```python
from build123d import *

# Parameters (mm, degrees)
F1_DEPTH = 6.5
F3_D     = 8.3


with BuildPart() as f1:
    # F0 (on Top) → F1 (new body)
    with BuildSketch(Plane.XY):
        Polygon((120, -32.1539030917), (0, 0), (-120, -32.1539030917), (-120, -156.3870447409), (0, -124.2331416492), (120, -156.3870447409), align=None)
    extrude(amount=F1_DEPTH)

    # F3 (through all)
    with Locations(Plane.XY.offset(6.5)):
        with Locations((-90, -44.820950927), (-41.7037086855, -31.8799986719), (-79.6472381959, -83.4579839786), (-31.3509468814, -70.5170317234), (-69.2944763918, -122.0950170301), (41.7037086855, -31.8799986719), (90, -44.820950927), (79.6472381959, -83.4579839786), (69.2944763918, -122.0950170301), (31.3509468814, -70.5170317234)):
            Hole(F3_D / 2)


solid = f1.part
```
Verification items for the finished model (mm, model axes). A direction names the side the tool comes from. Give positions to 0.01 mm unless a question says otherwise; leave off trailing zeros. Order: outer loops, then holes, each group sorted by start corner. A loop starts at its lowest first (then second) coordinate and runs counter-clockwise, first axis right, second up. Notation, with made-up numbers: M 13.5,40.25 L 30.5,40.25 A18 cw 30.5,55.25 Z; hole C 49,-10.75 d9. An arc over 180 degrees is marked long. Answer in a Markdown table with one row per item. Add a question column.
Item 1: Tool access check on faces 1 (the flat face through (59.16, -140.085, 3.204)), 2 (the cylindrical face through (-37.558, -31.698, 3.204)). Record the directions out of +Z, -Z, +X, -X, +Y, -Y that give a thin tool (end or side, any length) a straight path to the whole face; none if there is none.
Item 2: Section check C-C, the plane x = -59. Enter the section's corners in (y, z), and give its area (3 significant figures).
Item 3: Section check A-A, the plane x = -90.5. Enter the section's corners in (y, z), and give its area (3 significant figures).
Item 4: Scan lines: probe 1 along X at (y, z) = (-74, 4.75); probe 2 along X at (y, z) = (-124, 0.5); probe 3 along Y at (x, z) = (-73, 6). Record each from-to range of solid material in increasing order. Write a range as from..to.
Item 5: Section check B-B, the plane z = 3.5. State how many separate pieces and enclosed holes the cut face has, and give its area (3 significant figures).
Item 6: Mould release check, pull along X, two halves, no side actions. Record for faces 3 (the cylindrical face through (29.44, -74.2, 3.2)), 4 (the flat face through (-59.16, -15.85, 3.2)), 5 (the flat face through (-2, -77, 6.5)): released by +X, released by -X, zero draft, split by the parting line, or undercut.
Item 7: Gauge pin test, flat ends, axial feed: pin 1 (7.5 mm diameter, centred on x = 69.29, y = -122.1, fed in from -Z); pin 2 (1 mm diameter, centred on x = -50.5, z = 2.5, fed in from -Y). Record the tip position at first contact, or that the pin passes through.
Filled sheet:
| question | item | result |
|---|---|---|
| 1 | face 1 | +Z, -Z, -Y |
| 1 | face 2 | +Z, -Z |
| 2 | outline | M -140.04,0 L -15.81,0 L -15.81,6.5 L -140.04,6.5 Z |
| 2 | area | 808 mm^2 |
| 3 | outline | M -148.48,0 L -48.94,0 L -48.94,6.5 L -148.48,6.5 Z; M -40.7,0 L -24.25,0 L -24.25,6.5 L -40.7,6.5 Z |
| 3 | area | 754 mm^2 |
| 4 | probe 1 | x = -120..-33.61, -29.09..29.09, 33.61..120 |
| 4 | probe 2 | x = -120..-72.98, -65.61..65.61, 72.98..120 |
| 4 | probe 3 | y = -143.79..-123.96, -120.23..-19.56 |
| 5 | separate pieces | 1 |
| 5 | enclosed holes | 10 |
| 5 | area | 29,300 mm^2 |
| 6 | face 3 | undercut |
| 6 | face 4 | released by -X |
| 6 | face 5 | zero draft |
| 7 | pin 1 | passes through |
| 7 | pin 2 | stops at y = -137.9 |
